Print and shaded views of the part. All mm, measured from the part's lowest x, y and z. A direction names the side the tool comes from. Round coordinates to 2 decimals unless told otherwise and drop trailing zeros. Order: outer loops, then holes, each group sorted by start corner. A loop starts at its lowest first (then second) coordinate and runs counter-clockwise, first axis right, second up. Notation, with made-up numbers: M -4,71.25 L 26,71.25 A22 ccw 26,95.25 Z; hole C 35.5,-1 d8. An arc over 180 degrees is marked long. Write each question's results on one line, items separated by ' | '. Start each with the question number.
1. Band-saw the part on A-A, the plane x = 19.5. List the corners of the cut face in (y, z), then the cut area to 3 significant figures.
2. Band-saw the part on B-B, the plane z = 6. Give the number of separate pieces and of enclosed holes in the cut face, then the cut area to 3 significant figures.
3. Two-plate mould, pull along X, no slides. Class the marked faces 1, 2, 3 and 4: +X half, -X half, draft (parallel to the pull), parting line (faces both ways), or undercut.
4. Band-saw the part on C-C, the plane y = 5.75. List the corners of the cut face in (x, z), then the cut area to 3 significant figures.
5. Drop flat-ended pins along their axis: pin 1 Ø3 at (x, z) = (5, 6) entering from +Y; pin 2 Ø6 at (x, z) = (42, 10) entering from +Y; pin 3 Ø2.5 at (y, z) = (21.5, 3) entering from -X; pin 4 Ø6 at (x, z) = (9, 5) entering from -Y. Give the stop position or say it passes through.
6. Which spindle directions (+Z, -Z, +X, -X, +Y, -Y) get a long thin tool onto all of the face, cutting with end or side? Do the marked faces 5, 6, 7, 8 and 9. Say none if no direction does.
7. Band-saw the part on D-D, the plane z = 11.25. List the corners of the cut face in (x, y).
8. Probe L1, parallel to X at y = 5.5, z = 9.25; L2, parallel to Y at x = 20.5, z = 7; L3, parallel to Y at x = 20, z = 4. List the from-to ranges inside material, lowest first. Write a range as [from, to].
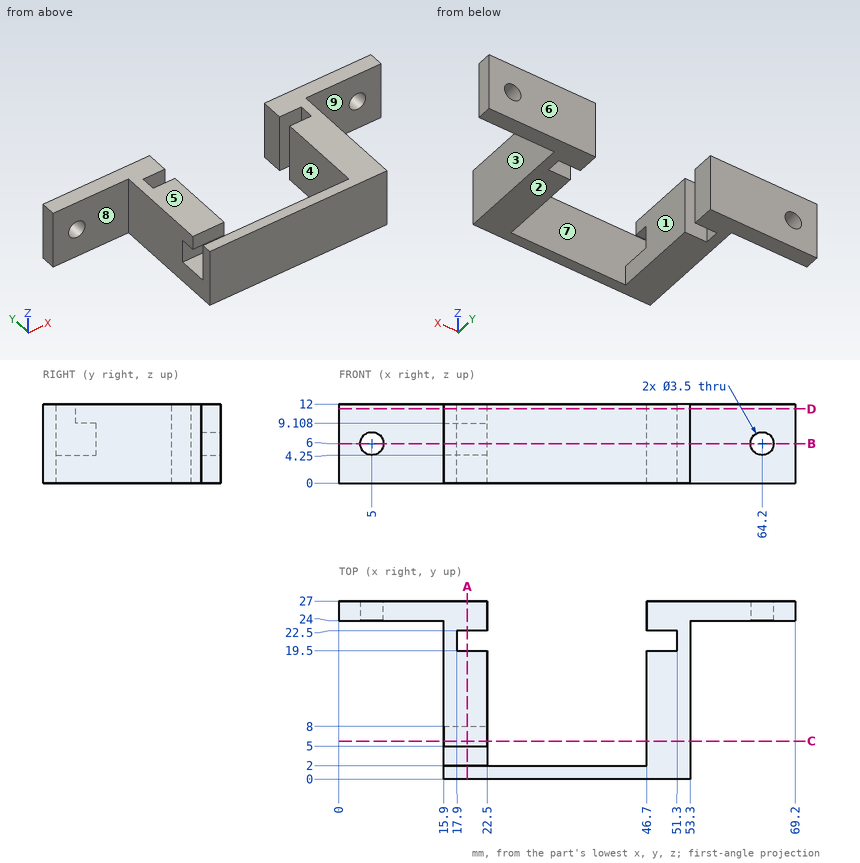
Solution:
1) outline: M 0,0 L 19.5,0 L 19.5,12 L 5,12 L 5,9.11 L 8,9.11 L 8,4.25 L 2,4.25 L 2,12 L 0,12 Z; M 22.5,0 L 27,0 L 27,12 L 22.5,12 Z | area: 250 mm^2
2) separate pieces: 4 | enclosed holes: 0 | area: 412 mm^2
3) face 1: undercut | face 2: draft | face 3: +X half | face 4: undercut
4) outline: M 15.9,0 L 22.5,0 L 22.5,4.25 L 15.9,4.25 Z; M 15.9,9.11 L 22.5,9.11 L 22.5,12 L 15.9,12 Z; M 46.7,0 L 53.3,0 L 53.3,12 L 46.7,12 Z | area: 126 mm^2
5) pin 1: through | pin 2: y = 2 | pin 3: x = 15.9 | pin 4: y = 24
6) face 5: +Z, +X, -X, +Y, -Y | face 6: +Z, -Z, +X, -X, +Y | face 7: +Z | face 8: +Z, -Z, -X, -Y | face 9: +Z, -Z, +X, -Y
7) outline: M 0,24 L 15.9,24 L 15.9,5 L 22.5,5 L 22.5,19.5 L 17.9,19.5 L 17.9,22.5 L 22.5,22.5 L 22.5,27 L 0,27 Z; M 15.9,0 L 53.3,0 L 53.3,24 L 69.2,24 L 69.2,27 L 46.7,27 L 46.7,22.5 L 51.3,22.5 L 51.3,19.5 L 46.7,19.5 L 46.7,2 L 15.9,2 Z
8) L1: [15.9, 22.5], [46.7, 53.3] | L2: [0, 2], [8, 19.5], [22.5, 27] | L3: [0, 19.5], [22.5, 27]
